Autodesk Inventor part; units mm, degrees
ref_plane "YZ Plane" through (0, 0, 0) normal (1, 0, 0) x (0, 1, 0)
ref_plane "XZ Plane" through (0, 0, 0) normal (0, 1, 0) x (-1, 0, 0)
ref_plane "XY Plane" through (0, 0, 0) normal (0, 0, 1) x (1, 0, 0)
sketch "Boceto1" plane through (0, 0, 0) normal (0, 1, 0) x (-1, 0, 0)
  line L0 (-60, 85) -> (-60, -85)
  line L1 (-60, -85) -> (60, -85)
  line L2 (60, -85) -> (60, 85)
  line L3 (-30, 85) -> (-30, 25)
  line L4 (-30, 25) -> (30, 25)
  line L5 (30, 25) -> (30, 85)
  line L6 (60, 85) -> (30, 85)
  line L7 (-30, 85) -> (-60, 85)
  point P0 (0, 0)
  dimension "d0" = 120
  dimension "d1" = 170
  dimension "d2" = 60
  dimension "d4" = 60
  dimension "d5" = 60
  dimension "d6" = 30
  dimension "d11" = 60
  dimension "d12" = 85
extrude "Extrusión1" add sketch "Boceto1" along normal blind 1
sketch "Boceto2" plane through (0, 1, 0) normal (0, 1, 0) x (1, 0, 0)
  line L0 (-60, 85) -> (-55, 85)
  line L1 (-59, 84) -> (-59, -85)
  line L2 (-59, -85) -> (-60, -85)
  line L3 (-60, -85) -> (-60, 85)
  line L4 (60, -85) -> (60, 85)
  line L5 (-60, 85) -> (60, 85)
  line L6 (60, 85) -> (60, 84)
  line L7 (59, 84) -> (-59, 84)
  line L8 (-60, 20) -> (-60, 85)
  line L9 (60, 85) -> (55, 85)
  line L10 (59, 84) -> (59, -85)
  line L11 (59, -85) -> (60, -85)
  line L12 (60, -85) -> (60, 85)
  line L13 (-30, -25) -> (30, -25)
  point P0 (0, 0)
  point P1 (60, -85)
  point P2 (60, 85)
  dimension "d15" = 1
  dimension "d17" = 1
  dimension "d18" = 1
  dimension "d22" = 170
  dimension "d23" = 1
  dimension "d24" = 170
  dimension "d57" = 0
  dimension "d58" = 0
  dimension "d59" = 5
  dimension "d60" = 115
  dimension "d61" = 115
  dimension "d62" = 0
  dimension "d63" = 0
  dimension "d64" = 0
extrude "Extrusión2" add sketch "Boceto2" along normal blind 45
sketch "Sketch37" plane through (0, 1, 0) normal (0, 1, 0) x (1, 0, 0)
  line L0 (-30, -25) -> (30, -25)
  line L1 (30, -24) -> (-30, -24)
  line L2 (-31, -25) -> (-31, -40)
  line L3 (-31, -40) -> (-30, -40)
  line L4 (-30, -40) -> (-30, -25)
  line L5 (30, -25) -> (30, -85)
  line L6 (31, -25) -> (31, -40)
  line L7 (31, -40) -> (30, -40)
  line L8 (30, -40) -> (30, -25)
  line L9 (-31, -25) -> (-31, -24)
  line L10 (-31, -24) -> (-30, -24)
  line L11 (30, -24) -> (31, -24)
  line L12 (31, -24) -> (31, -25)
  point P0 (0, 0)
  dimension "d127" = 1
  dimension "d129" = 1
  dimension "d130" = 90
  dimension "d131" = 16
  dimension "d132" = 15
  dimension "d133" = 0
  dimension "d134" = 60
  dimension "d135" = 15
  dimension "d136" = 15
extrude "Extrusion26" add sketch "Sketch37" along normal blind 30
sketch "Sketch39" plane through (0, 1, 0) normal (0, 1, 0) x (1, 0, 0)
  line L0 (-51, -45) -> (-40, -45)
  line L1 (-40, -45) -> (-40, -78)
  line L2 (-40, -78) -> (-51, -78)
  line L3 (-51, -78) -> (-51, -45)
  line L4 (-30, -85) -> (-30, -40)
  line L5 (-59, -85) -> (-30, -85)
  point P0 (0, 0)
  dimension "d139" = 11
  dimension "d140" = 33
  dimension "d141" = 10
  dimension "d142" = 7
extrude "Extrusion27" add sketch "Sketch39" along normal blind 1
sketch "Sketch42" plane through (-59, 1, 85) normal (1, 0, 0) x (0, 0, -1)
  line L0 (0, 45) -> (169, 45)
  line L1 (0, 0) -> (45, 0) construction
  line L2 (45, 0) -> (45, 45) construction
  line L3 (45, 45) -> (0, 45) construction
  line L4 (0, 45) -> (0, 0) construction
  line L5 (0, 0) -> (169, 0)
  line L6 (169, 0) -> (169, 45)
  line L7 (0, 45) -> (169, 45)
  line L8 (0, 0) -> (0, 45)
  line L9 (0, -1) -> (0, 0)
  line L10 (170, -1) -> (0, -1)
  line L11 (170, 45) -> (170, -1)
  line L12 (169, 45) -> (170, 45)
  line L13 (0, 0) -> (45, 45)
  line L14 (0, 45) -> (0, 0)
  line L15 (0, -1) -> (0, 45)
  point P0 (85, -1)
  dimension "d159" = 45
extrude "Extrusion30" cut sketch "Sketch42" against normal blind 33.25 contours L0 L13 L8
sketch "Sketch43" plane through (-59, 1, -84) normal (1, 0, 0) x (0, 0, -1)
  line L0 (0, 0) -> (-169, 0)
  line L1 (-159.5434, 0) -> (-159.5434, 11.2545) construction
  line L2 (-169, 0) -> (-124, 45)
  line L3 (-159.5434, 9.4566) -> (-169, 0)
  line L4 (-169, 0) -> (-168, 0)
  line L5 (-168, 0) -> (-159.0434, 8.9566)
  line L6 (-159.0434, 8.9566) -> (-159.5434, 9.4566)
  point P0 (-84, -1)
  dimension "d162" = 1
extrude "Extrusion31" add sketch "Sketch43" along normal blind 29
sketch "Sketch45" plane through (-30, 0, 85) normal (1, 0, 0) x (0, 0, -1)
  line L0 (9.4566, 10.4566) -> (0, 1)
  line L1 (4.7283, 5.7283) -> (9.4566, 10.4566)
  line L2 (9.4566, 10.4566) -> (9.9566, 9.9566)
  line L3 (9.4566, 10.4566) -> (9.9566, 9.9566)
  line L4 (9.9566, 9.9566) -> (5.2283, 5.2283)
  line L5 (1, 1) -> (9.9566, 9.9566)
  line L6 (4.7283, 5.7283) -> (5.2283, 5.2283)
  point P0 (85, 0)
extrude "Extrusion33" cut sketch "Sketch45" against normal blind 16
sketch "Sketch46" plane through (0, 2, 0) normal (0, 1, 0) x (1, 0, 0)
  line L0 (-40, -78) -> (-40, -45)
  line L1 (-40, -45) -> (-41, -45)
  line L2 (-41, -45) -> (-41, -78)
  line L3 (-41, -78) -> (-40, -78)
  line L4 (-40, -78) -> (-40, -45)
  point P0 (0, 0)
  dimension "d169" = 1
extrude "Extrusion34" add sketch "Sketch46" along normal blind 45
sketch "Sketch47" plane through (-40, 1, 78) normal (1, 0, 0) x (0, 0, -1)
  line L0 (5, 43) -> (28, 43) construction
  line L1 (0, 0) -> (0, 46)
  line L2 (5, 14) -> (28, 14) construction
  line L3 (0, 46) -> (33, 46)
  circle A0 centre (5, 43) radius 1.5
  circle A1 centre (28, 43) radius 1.5
  circle A2 centre (5, 14) radius 1.5
  circle A3 centre (28, 14) radius 1.5
  point P0 (78, -1)
  dimension "d172" = 23
  dimension "d173" = 5
  dimension "d174" = 29
  dimension "d175" = 3
  dimension "d176" = 3
  dimension "d177" = 3
  dimension "d178" = 3
  dimension "d179" = 3
extrude "Extrusion35" cut sketch "Sketch47" against normal blind 1
sketch "Sketch50" plane through (60, 0, 85) normal (1, 0, 0) x (0, 0, -1)
  line L0 (0, 1) -> (45, 46)
  line L1 (0, 1) -> (45, 46)
  line L2 (169, 46) -> (0, 46)
  line L3 (45, 46) -> (0, 46)
  line L4 (0, 46) -> (0, 1)
  line L5 (0, 0) -> (0, 46)
  point P0 (85, 0)
extrude "Extrusion36" cut sketch "Sketch50" against normal blind 1
sketch "Sketch51" plane through (59, 1, -84) normal (-1, 0, 0) x (0, 0, 1)
  line L0 (124, 45) -> (169, 0)
  line L1 (124, 45) -> (169, 0)
  line L2 (169, 0) -> (168, 0)
  line L3 (169, 0) -> (0, 0)
  line L4 (168, 0) -> (123.5, 44.5)
  line L5 (0, 45) -> (124, 45)
  line L6 (123.5, 44.5) -> (124, 45)
  point P0 (84, -1)
  dimension "d185" = 1
extrude "Extrusion37" add sketch "Sketch51" along normal blind 29
sketch "Sketch52" plane through (-60, 0, -85) normal (-1, 0, 0) x (0, 0, 1)
  line L0 (169, 1) -> (1, 1)
  line L1 (16, 1) -> (26, 1)
  line L2 (26, 1) -> (26, 11)
  line L3 (26, 11) -> (16, 11)
  line L4 (16, 11) -> (16, 1)
  line L5 (1, 1) -> (1, 46)
  point P0 (85, 0)
  point P1 (26, 1)
  dimension "d188" = 10
  dimension "d189" = 10
  dimension "d190" = 15
extrude "Extrusion38" cut sketch "Sketch52" against normal blind 120
sketch "Sketch53" plane through (0, 1, 0) normal (0, 1, 0) x (1, 0, 0)
  line L0 (-59, 69) -> (-44, 69)
  line L1 (-44, 69) -> (-44, 71)
  line L2 (-44, 71) -> (-59, 71)
  line L3 (-59, 71) -> (-59, 69)
  line L4 (-59, 59) -> (-59, -84)
  line L5 (-59, 59) -> (-44, 59)
  line L6 (-44, 59) -> (-44, 57)
  line L7 (-44, 57) -> (-59, 57)
  line L8 (-59, 57) -> (-59, 59)
  line L9 (59, 69) -> (59, 84)
  line L10 (59, 69) -> (44, 69)
  line L11 (44, 69) -> (44, 71)
  line L12 (44, 71) -> (59, 71)
  line L13 (59, 71) -> (59, 69)
  line L14 (59, 69) -> (59, 59)
  line L15 (59, 59) -> (44, 59)
  line L16 (44, 59) -> (44, 57)
  line L17 (44, 57) -> (59, 57)
  line L18 (59, 57) -> (59, 59)
  point P0 (0, 0)
  dimension "d193" = 15
  dimension "d194" = 2
  dimension "d195" = 15
  dimension "d196" = 2
  dimension "d197" = 15
extrude "Extrusion39" add sketch "Sketch53" along normal blind 10
properties part number "Chasisneww"
Geometry: final body of the model. Coordinates: model frame, mm. A direction names the side the tool comes from. Coordinates: 2 decimals unless noted, no trailing zeros. Order: outer loops, then holes, each group sorted by start corner. A loop starts at its lowest first (then second) coordinate and runs counter-clockwise, first axis right, second up.
Item 1: Contact query for flat-ended pins moving along their axis: P1, Ø5, axis at x = 22, y = 36.5, coming from the +Z side; P2, Ø8, axis at x = 37, y = 18, coming from the +Z side; P3, Ø6, axis at x = 29.5, y = 18.5, coming from the +Z side; P4, Ø1.5, axis at x = -27.5, z = 28.5, coming from the +Y side. Output: stop coordinate, or through.
Answer:
P1: stops at z = -84
P2: stops at z = 72
P3: stops at z = 70.46
P4: passes through
Item 2: Access query for faces 1 (the face through (-30, 14, 37)), 2 (the face through (-40.6, 18.8, 45)), 3 (the face through (45, 24, 62)). Directions: +Z, -Z, +X, -X, +Y, -Y. A direction counts if a zero-diameter tool reaches every point of the face in a straight line with its end or side. Return the directions, or none.
Answer:
face 1: +Z, +Y, -Y
face 2: +Y
face 3: +Z, +X, +Y
Item 3: Section query D-D (x = 27). Output: boundary loops of the cut face in (y, z), then the cut area to 3 significant figures.
Answer:
outline: (0, -85) - (46, -85) - (46, -84) - (1, -84) - (1, 24) - (31, 24) - (31, 25) - (0, 25) - close
area: 185 mm2
Item 4: Draft query along Z for faces 4 (the face through (-50, 8, 78)), 5 (the face through (0, 16, 24)), 6 (the face through (1, 0, -18)). Return one class per face: released by +Z, released by -Z, zero draft, split by the parting line, or undercut.
Answer:
face 4: released by +Z
face 5: undercut
face 6: zero draft
Item 5: Section query A-A (y = 22.5). Output: boundary loops of the cut face in (x, z).
Answer:
outline: (-60, -85) - (60, -85) - (60, 63.5) - (30, 63.5) - (30, 62.5) - (59, 62.5) - (59, -84) - (-59, -84) - (-59, 63.5) - (-60, 63.5) - close; (-41, 45) - (-40, 45) - (-40, 78) - (-41, 78) - close; (-31, 24) - (31, 24) - (31, 40) - (30, 40) - (30, 25) - (-30, 25) - (-30, 40) - (-31, 40) - close
Item 6: Section query C-C (y = 38). Output: boundary loops of the cut face in (x, z).
Answer:
outline: (-60, -85) - (60, -85) - (60, 48) - (30, 48) - (30, 47) - (59, 47) - (59, -84) - (-59, -84) - (-59, 48) - (-60, 48) - close; (-41, 45) - (-40, 45) - (-40, 78) - (-41, 78) - close
Item 7: Section query B-B (z = -2.5). Output: boundary loops of the cut face in (x, y).
Answer:
outline: (-60, 0) - (60, 0) - (60, 46) - (59, 46) - (59, 1) - (-59, 1) - (-59, 46) - (-60, 46) - close
Item 8: Material intervals for line 1 along Y through (x, z) = (-40.35, 73); line 2 along X through (y, z) = (5, 39); line 3 along X through (y, z) = (3, 22), sorted ascending.
Answer:
line 1: y = 0 to 13.5, 16.5 to 42.5, 45.5 to 47
line 2: x = -60 to -59, -31 to -30, 30 to 31, 59 to 60
line 3: x = -60 to -59, 59 to 60
